Geometry: final body of the model. Coordinates: model frame, mm. Face numbers are marked on the shaded views. Round coordinates to 2 decimals unless told otherwise and drop trailing zeros. Loops run counter-clockwise (first coordinate to the right, second up) from the corner with the lowest first, then second, coordinate; pieces in that order, holes last. Notation, with made-up numbers: (63.25, -15.75) - (99.25, -15.75) arc R37 ccw to (99.25, 21.25) - close; hole circle Ø10 at (-10.5, 1.25). An arc over 180 degrees is marked (long way). Return JSON: item names as keys, results as strings. Group by question number.
1. Section D-D on z = 13. Count the separate pieces of the cut face and the enclosed holes in it, and give its area (3 significant figures).
2. Section A-A on y = 25.5. Return loops of the section in (x, z), and give its area (3 significant figures).
3. Section B-B on x = 133.5. Return loops of the section in (y, z).
4. Material intervals for probe 1 along X at (y, z) = (-2.5, 10.9); probe 2 along Y at (x, z) = (135, 11.55); probe 3 along X at (y, z) = (-11.5, 12.15), sorted ascending.
5. First-contact query: pin 1 Ø1.1 at (x, y) = (34, -43) entering from +Z; pin 2 Ø1.5 at (x, z) = (107.5, 13) entering from +Y; pin 3 Ø1.9 at (x, y) = (32.5, 43.5) entering from +Z. Flat tips, straight axial feed; report the tip coordinate or a pass-through.
6. Section C-C on y = 13. Return loops of the section in (x, z), and give its area (3 significant figures).
7. Draft query along Y for the marked faces 1 and 2. Return one class per face: +Y half, -Y half, draft (parallel to the pull), parting line (faces both ways), or undercut.
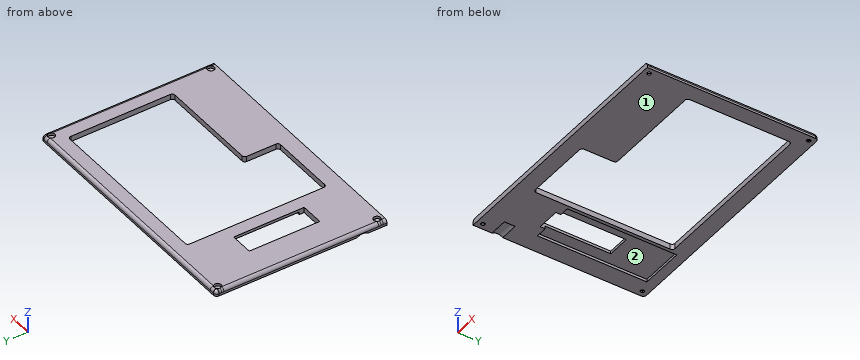
from build123d import *

# Parameters (mm, degrees)
SKETCH057_W                       = 140
SKETCH057_H                       = 93.9
PAD006_DEPTH                      = 3
SKETCH058_W                       = 12.5
SKETCH058_H                       = 38.6472
POCKET043_DEPTH                   = 3
SKETCH059_W                       = 24
SKETCH059_H                       = 60
POCKET044_DEPTH                   = 1.5
SKETCH060_R                       = 1.05
POCKET045_DEPTH                   = 3.001
SKETCH061_R                       = 1.9
POCKET046_DEPTH                   = 1.4
CHAMFER002_1_ANGLE                = 45
CHAMFER002_1_SIZE                 = 0.843
CHAMFER002_2_ANGLE                = 45
CHAMFER002_2_SIZE                 = 0.843
CHAMFER002_3_ANGLE                = 45
CHAMFER002_3_SIZE                 = 0.843
CHAMFER002_4_ANGLE                = 45
CHAMFER002_4_SIZE                 = 0.843
FILLET007_R                       = 1.5
SKETCH062_R                       = 4.85
POCKET047_DEPTH                   = 10
FILLET008_R                       = 1.8
BODY005_PLACEMENT_ANGLE           = 180
PART_MIRRORING001_PLACEMENT_ANGLE = 180


with BuildPart() as top002:
    # Sketch057 (on XY_Plane154 of Origin626) → Pad006 (new body)
    with BuildSketch(Plane.XY):
        Rectangle(SKETCH057_W, SKETCH057_H)
    extrude(amount=PAD006_DEPTH)

    # Sketch058 (on Face6 of Pad006) → Pocket043 (cut)
    with BuildSketch(Plane.XY.offset(3)):
        Polygon((-61.3, 38.25), (-61.3, -19.25), (-4.3, -19.25), (-4.3, -38.25), (34.2, -38.25), (34.2, 38.25), align=None)
        with Locations((47.48708, -1.86296)):
            Rectangle(SKETCH058_W, SKETCH058_H)
    extrude(amount=-POCKET043_DEPTH, mode=Mode.SUBTRACT)

    # Sketch059 (on Face4 of Pocket043) → Pocket044 (cut)
    with BuildSketch(Plane(origin=(0, 0, 0), x_dir=(1, 0, 0), z_dir=(0, 0, -1))):
        with Locations((48, -11.55)):
            Rectangle(SKETCH059_W, SKETCH059_H)
    extrude(amount=-POCKET044_DEPTH, mode=Mode.SUBTRACT)

    # Sketch060 (on Face5 of Pocket044) → Pocket045 (cut, through all)
    with BuildSketch(Plane.XY.offset(3)):
        with Locations((66.75, 43.7)):
            Circle(SKETCH060_R)
        with Locations((66.75, -43.7)):
            Circle(SKETCH060_R)
        with Locations((-66.75, -43.7)):
            Circle(SKETCH060_R)
        with Locations((-66.75, 43.7)):
            Circle(SKETCH060_R)
    extrude(amount=-POCKET045_DEPTH, mode=Mode.SUBTRACT)

    # Sketch061 (on Face5 of Pocket045) → Pocket046 (cut)
    with BuildSketch(Plane.XY.offset(3)):
        with Locations((-66.75, 43.7)):
            Circle(SKETCH061_R)
        with Locations((66.75, 43.7)):
            Circle(SKETCH061_R)
        with Locations((-66.75, -43.7)):
            Circle(SKETCH061_R)
        with Locations((66.75, -43.7)):
            Circle(SKETCH061_R)
    extrude(amount=-POCKET046_DEPTH, mode=Mode.SUBTRACT)

    # Chamfer002 1
    chamfer002_1_edges = [top002.edges().sort_by_distance(p)[0] for p in [
        (-67.8, 43.7, 1.6),
    ]]
    chamfer002_1_side = top002.faces().sort_by_distance((-67.8, 43.7, 0.8))[0]
    chamfer(chamfer002_1_edges, length=CHAMFER002_1_SIZE, angle=CHAMFER002_1_ANGLE, reference=chamfer002_1_side)

    # Chamfer002 2
    chamfer002_2_edges = [top002.edges().sort_by_distance(p)[0] for p in [
        (65.7, -43.7, 1.6),
    ]]
    chamfer002_2_side = top002.faces().sort_by_distance((65.7, -43.7, 0.8))[0]
    chamfer(chamfer002_2_edges, length=CHAMFER002_2_SIZE, angle=CHAMFER002_2_ANGLE, reference=chamfer002_2_side)

    # Chamfer002 3
    chamfer002_3_edges = [top002.edges().sort_by_distance(p)[0] for p in [
        (-67.8, -43.7, 1.6),
    ]]
    chamfer002_3_side = top002.faces().sort_by_distance((-67.8, -43.7, 0.8))[0]
    chamfer(chamfer002_3_edges, length=CHAMFER002_3_SIZE, angle=CHAMFER002_3_ANGLE, reference=chamfer002_3_side)

    # Chamfer002 4
    chamfer002_4_edges = [top002.edges().sort_by_distance(p)[0] for p in [
        (65.7, 43.7, 1.6),
    ]]
    chamfer002_4_side = top002.faces().sort_by_distance((65.7, 43.7, 0.8))[0]
    chamfer(chamfer002_4_edges, length=CHAMFER002_4_SIZE, angle=CHAMFER002_4_ANGLE, reference=chamfer002_4_side)

    # Fillet007
    fillet007_edges = [top002.edges().sort_by_distance(p)[0] for p in [
        (-4.3, -38.25, 1.5),
        (34.2, -38.25, 1.5),
        (34.2, 38.25, 1.5),
        (-61.3, 38.25, 1.5),
        (-61.3, -19.25, 1.5),
        (-4.3, -19.25, 1.5),
    ]]
    fillet(fillet007_edges, radius=FILLET007_R)

    # Sketch062 (on Face16 of Fillet007) → Pocket047 (cut)
    with BuildSketch(Plane.YZ.offset(70)):
        with Locations((-33.64, -3.85)):
            Circle(SKETCH062_R)
    extrude(amount=-POCKET047_DEPTH, mode=Mode.SUBTRACT)

    # Fillet008
    fillet008_edges = [top002.edges().sort_by_distance(p)[0] for p in [
        (70, 0, 3),
        (0, 46.95, 3),
        (70, 46.95, 1.5),
        (-70, 46.95, 1.5),
        (-70, 0, 3),
    ]]
    fillet(fillet008_edges, radius=FILLET008_R)


with BuildPart() as top002_1:
    # Body005 placement: moved
    add(top002.part.moved(Location((150, 0, 2.9))).rotate(Axis((150, 0, 2.9), (0, 1, 0)), BODY005_PLACEMENT_ANGLE))


with BuildPart() as part_mirroring001:
    # Part__Mirroring001: instance of Top002
    add(top002_1.part.mirror(Plane(origin=(0, 0, 0), x_dir=(0, -1, 0), z_dir=(1, 0, 0))))


with BuildPart() as part_mirroring001_1:
    # Part__Mirroring001 placement: moved
    add(part_mirroring001.part.moved(Location((-50, 0, 13.4))).rotate(Axis((-50, 0, 13.4), (0, 1, 0)), PART_MIRRORING001_PLACEMENT_ANGLE))


solid = part_mirroring001_1.part
Taken from the geometry:
{
 "1": {"separate pieces": "1", "enclosed holes": "6", "area": "6,220 mm2"},
 "2": {"outline": "(30, 10.5) - (40, 10.5) - (40, 12) - (64, 12) - (64, 10.5) - (65.8, 10.5) - (65.8, 13.5) - (31.8, 13.5) arc R1.8 ccw to (30, 11.7) - close; (161.3, 10.5) - (170, 10.5) - (170, 11.7) arc R1.8 ccw to (168.2, 13.5) - (161.3, 13.5) - close", "area": "96.1 mm2"},
 "3": {"outline": "(-46.95, 10.5) - (-19.25, 10.5) - (-19.25, 13.5) - (-46.95, 13.5) - close; (38.25, 10.5) - (46.95, 10.5) - (46.95, 11.7) arc R1.8 ccw to (45.15, 13.5) - (38.25, 13.5) - close"},
 "4": {"probe 1": "30 to 40, 64 to 65.8, 161.3 to 170", "probe 2": "-46.95 to -19.25, 38.25 to 46.95", "probe 3": "30.06 to 46.26, 58.76 to 65.8, 161.3 to 169.94"},
 "5": {"pin 1": "z = 11.78", "pin 2": "y = 46.86", "pin 3": "z = 11.93"},
 "6": {"outline": "(30, 10.5) - (40, 10.5) - (40, 12) - (46.26, 12) - (46.26, 13.5) - (31.8, 13.5) arc R1.8 ccw to (30, 11.7) - close; (58.76, 12) - (64, 12) - (64, 10.5) - (65.8, 10.5) - (65.8, 13.5) - (58.76, 13.5) - close; (161.3, 10.5) - (170, 10.5) - (170, 11.7) arc R1.8 ccw to (168.2, 13.5) - (161.3, 13.5) - close", "area": "77.4 mm2"},
 "7": {"face 1": "draft", "face 2": "undercut"}
}
